Job drawing, mm, ordinate dimensions from the low corner. One solid piece. A direction names the side the tool comes from. Give positions to 0.01 mm unless a question says otherwise; leave off trailing zeros. Loops run counter-clockwise (first coordinate to the right, second up) from the corner with the lowest first, then second, coordinate; pieces in that order, holes last. Notation, with made-up numbers: M 64,78.25 L 120,78.25 A29 ccw 120,102.25 Z; hole C 70,-20 d10. An arc over 180 degrees is marked long. Answer as CSV lines item,"result".
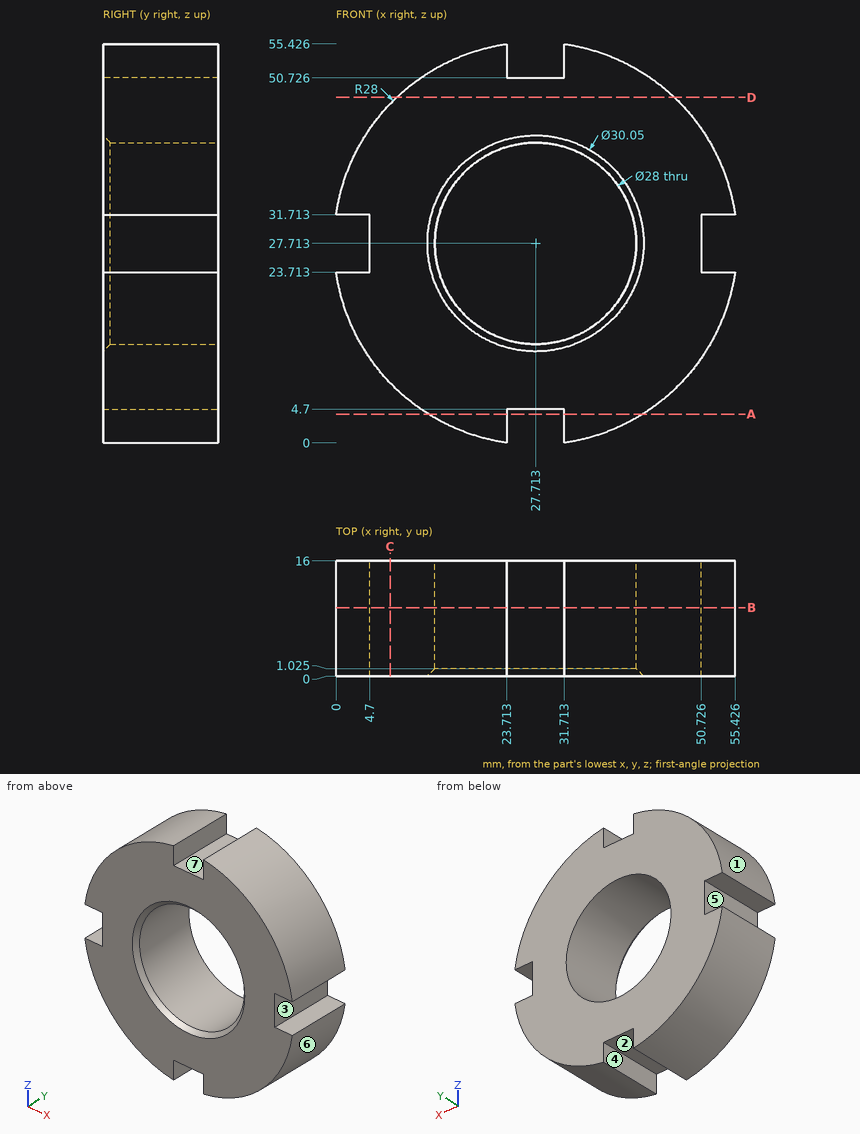
1) Mould opens along X. For the marked faces 1, 2, 3 and 4 say: +X half, -X half, draft (parallel to the pull), parting line (faces both ways), or undercut.
Answer below:
face 1,"-X half"
face 2,"undercut"
face 3,"+X half"
face 4,"undercut"
2) Band-saw the part on A-A on z = 4. Give the cut face in (x, y).
Answer below:
outline,"M 12.82,0 L 23.71,0 L 23.71,16 L 12.82,16 Z; M 31.71,0 L 42.6,0 L 42.6,16 L 31.71,16 Z"
3) Band-saw the part on D-D on z = 48. Give the cut face in (x, y) (1 decimal).
Answer below:
outline,"M 8.4,0 L 47,0 L 47,16 L 8.4,16 Z"
4) Band-saw the part on B-B on y = 9.5. Give the cut face in (x, z) (1 decimal), and give its area (3 significant figures).
Answer below:
outline,"M 0,23.7 A28 ccw 23.7,0 L 23.7,4.7 L 31.7,4.7 L 31.7,0 A28 ccw 55.4,23.7 L 50.7,23.7 L 50.7,31.7 L 55.4,31.7 A28 ccw 31.7,55.4 L 31.7,50.7 L 23.7,50.7 L 23.7,55.4 A28 ccw 0,31.7 L 4.7,31.7 L 4.7,23.7 Z; hole C 27.7,27.7 d28"
area,"1,690 mm^2"
5) Band-saw the part on C-C on x = 7.5. Give the cut face in (y, z).
Answer below:
outline,"M 0,8.34 L 16,8.34 L 16,47.09 L 0,47.09 Z"
6) Which spindle directions (+Z, -Z, +X, -X, +Y, -Y) get a long thin tool onto all of the face, cutting with end or side? Do the marked faces 5, 6 and 7. Say none if no direction does.
Answer below:
face 5,"-X, +Y, -Y"
face 6,"-Z, +X, +Y, -Y"
face 7,"+Z, +Y, -Y"
7) Drill centre lines: line 1 (Z direction, x = 19, y = 9.5) (1 decimal); line 2 (X direction, y = 7.25, z = 17.5) (1 decimal); line 3 (X direction, y = 8, z = 21) (1 decimal). Where is each one in solid material? Low to high. Write a range as from..to.
Answer below:
line 1,"z = 1.1..16.8, 38.7..54.3"
line 2,"x = 1.6..18.1, 37.3..53.8"
line 3,"x = 0.5..15.4, 40..54.9"
8) Flat gauge pins, fed straight in: pin 1 (4 mm diameter, centred on x = 27, y = 9.5, fed in from +Z); pin 2 (2.5 mm diameter, centred on y = 4.5, z = 52.5, fed in from +X); pin 3 (2.5 mm diameter, centred on y = 6, z = 29, fed in from -X). Where does each tip first touch, or does it go through?
Answer below:
pin 1,"stops at z = 50.73"
pin 2,"stops at x = 42.88"
pin 3,"stops at x = 4.7"
